Geometry: see drawing. Coordinates: mm, zero at the bounding-box minimum. A direction names the side the tool comes from. Give positions to 0.01 mm unless a question says otherwise; leave off trailing zeros. Order: outer loops, then holes, each group sorted by start corner. A loop starts at its lowest first (then second) coordinate and runs counter-clockwise, first axis right, second up. Notation, with made-up numbers: (63.5, 59.25) - (78.5, 59.25) arc R32 ccw to (78.5, 89.25) - close; hole circle Ø3 at (-23.5, -22). An arc over 180 degrees is marked (long way). Write item = value, one per line. Start each with the question number.
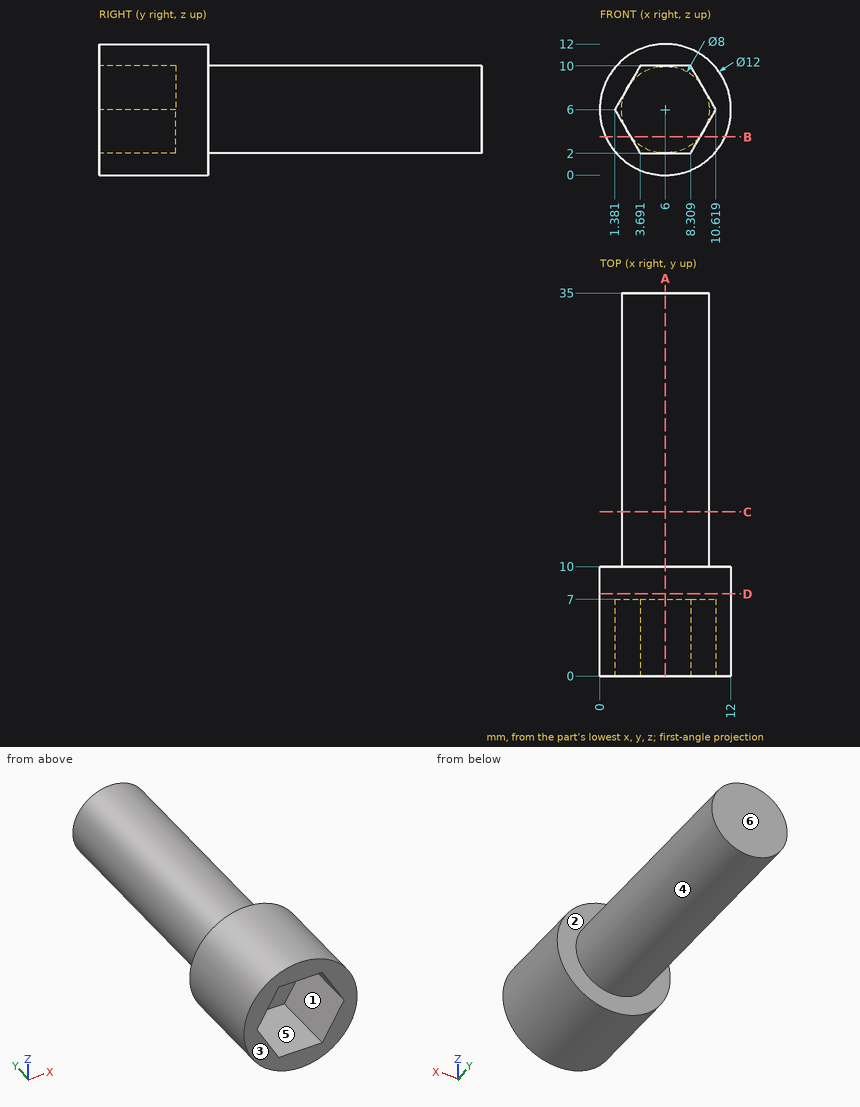
Q1. Pull-direction query (X, two-part tool) for the marked faces 4, 5 and 6; classes: +X half, -X half, draft (parallel to the pull), parting line (faces both ways), or undercut.
Q2. Section D-D, the plane y = 7.5. Return the cut outline in (x, z).
Q3. Section A-A, the plane x = 6. Return the cut outline in (y, z), then the cut area to 3 significant figures.
Q4. Set-up query: the marked faces 1, 2 and 3. Return all of +Z, -Z, +X, -X, +Y, -Y with unobstructed straight access to the full face (end or side cutting, diameter ignored); none if empty.
Q5. Section C-C, the plane y = 15. Return the cut outline in (x, z).
Q6. Section B-B, the plane z = 3.5. Return the cut outline in (x, y) (1 decimal), then the cut area to 3 significant figures.
Q7. Material intervals for line 1 along Y through (x, z) = (8.5, 7.5); line 2 along X through (y, z) = (3, 9.5) (1 decimal); line 3 along X through (y, z) = (3.5, 2.75) (1 decimal), sorted ascending. Write a range as from..to.
Q8. Contact query for flat-ended pins moving along their axis: pin 1 (6 mm diameter, centred on y = 16.5, z = 7.5, fed in from -X); pin 2 (3.5 mm diameter, centred on x = 6.5, y = 3, fed in from +Z); pin 3 (1.5 mm diameter, centred on y = 6, z = 7, fed in from +X) (1 decimal); pin 4 (3 mm diameter, centred on y = 6, z = 2, fed in from -X) (1 decimal). Output: stop coordinate, or through.
The answers:
q1.face_4 = parting line
q1.face_5 = undercut
q1.face_6 = draft
q2.outline = circle Ø12 at (6, 6)
q3.outline = (0, 0) - (10, 0) - (10, 2) - (35, 2) - (35, 10) - (10, 10) - (10, 12) - (0, 12) - (0, 10) - (7, 10) - (7, 2) - (0, 2) - close
q3.area = 264 mm²
q4.face_1 = -Y
q4.face_2 = +Y
q4.face_3 = +Z, -Z, +X, -X, -Y
q5.outline = circle Ø8 at (6, 6)
q6.outline = (0.5, 0) - (2.8, 0) - (2.8, 7) - (9.2, 7) - (9.2, 0) - (11.5, 0) - (11.5, 10) - (9.1, 10) - (9.1, 35) - (2.9, 35) - (2.9, 10) - (0.5, 10) - close
q6.area = 221 mm²
q7.line_1 = 7..35
q7.line_2 = 1.1..3.4, 8.6..10.9
q7.line_3 = 1..3.3, 8.7..11
q8.pin_1 = 2
q8.pin_2 = 12
q8.pin_3 = 12
q8.pin_4 = 0.5
